Autodesk Inventor part; units mm, degrees
ref_plane "YZ Plane" through (0, 0, 0) normal (1, 0, 0) x (0, 1, 0)
ref_plane "XZ Plane" through (0, 0, 0) normal (0, 1, 0) x (-1, 0, 0)
ref_plane "XY Plane" through (0, 0, 0) normal (0, 0, 1) x (1, 0, 0)
sketch "Sketch1" plane through (0, 0, 0) normal (0, 1, 0) x (-1, 0, 0)
  circle A0 centre (0, 0) radius 20
  dimension "d0" = 40
extrude "Extrusion1" add sketch "Sketch1" along normal blind 1000
sketch "Sketch2" plane through (0, 0, 0) normal (0, 0, 1) x (1, 0, 0)
  circle A0 centre (0, 190.0543) radius 1.5
  point P0 (0, 0)
  dimension "d3" = 3
extrude "Extrusion2" add sketch "Sketch2" along normal blind 25 and the other way blind 25
sketch "Sketch3" plane through (0, 190.0543, 25) normal (0, 0, 1) x (1, 0, 0)
  point P0 (0, -190.0543)
  point P1 (-0.0211, -0.0123)
hole "Hole1" at (-0.0211, 190.042, 25) direction (0, 0, -1) diameter 4 depth 51
sketch "Sketch4" plane through (0, 0, 0) normal (0, -1, 0) x (1, 0, 0)
  point P0 (0, 0)
  point P1 (0, 0)
hole "Hole2" at (0, 0, 0) direction (0, 1, 0) diameter 29 depth 906
thread "Thread2"
thread "Thread3"
properties part number "Tongkatttt" material "Aluminum 6061-AHC"
Part model, mm, in its own coordinate system. A direction names the side the tool comes from. Coordinates: 2 decimals unless noted, no trailing zeros. Write each loop counter-clockwise with the first axis right and the second up, starting at its lowest first coordinate (ties: lowest second). Pieces come first, ordered by that corner, then holes.
Item 1: Slice it at A-A (z = 0). Write the cut outline in (x, y), and give its area (3 significant figures).
Item 2: Probe line 1 (Z direction, x = 2, y = 275); line 2 (Z direction, x = -0.5, y = 756); line 3 (Y direction, x = -0.5, z = -3.5). List the from-to ranges inside material, lowest first.
Item 3: Which spindle directions (+Z, -Z, +X, -X, +Y, -Y) get a long thin tool onto all of the face, cutting with end or side? Do faces 4 (the face through (-10.3, 0, 10.5)), 5 (the face through (0, 906, 0)). Say none if no direction does.
Item 4: Slice it at B-B (y = 423.5). Write the cut outline in (x, z), and give its area (3 significant figures).
Item 5: Pin check, flat tips, straight feed: pin 1 (3 mm diameter, centred on y = 197.5, z = 5, fed in from +X); pin 2 (8 mm diameter, centred on x = -2.5, z = 7.5, fed in from -Y); pin 3 (4 mm diameter, centred on y = 632.5, z = -3.5, fed in from +X). Stop position of each tip, or through.
Item 6: Mould opens along X. For faces 1 (the face through (4.336, 493, 19.524)), 2 (the face through (12.864, 459.342, -6.691)), 3 (the face through (0, 1000, 0)) say: released by +X, released by -X, zero draft, split by the parting line, or undercut.
Item 7: Slice it at C-C (y = 921). Write the cut outline in (x, z).
Results found:
1. outline: (-20, 0) - (-14.5, 0) - (-14.5, 906) - (14.5, 906) - (14.5, 0) - (20, 0) - (20, 1000) - (-20, 1000) - close
1. area: 13,700 mm2
2. line 1: z = -19.9 to -14.36, 14.36 to 19.9
2. line 2: z = -19.99 to -14.49, 14.49 to 19.99
2. line 3: y = 906 to 1000
3. face 4: +Z, -Z, +X, -X, -Y
3. face 5: -Y
4. outline: circle Ø40 at (0, 0); hole circle Ø29 at (0, 0)
4. area: 596 mm2
5. pin 1: stops at x = 19.69
5. pin 2: stops at y = 906
5. pin 3: stops at x = 19.94
6. face 1: split by the parting line
6. face 2: undercut
6. face 3: zero draft
7. outline: circle Ø40 at (0, 0)
